For this review, take the finished solid that the model builds, in its own axes (mm). A direction names the side the tool comes from. Give positions to 0.01 mm unless a question says otherwise; leave off trailing zeros. Write each loop counter-clockwise with the first axis right and the second up, starting at its lowest first coordinate (ties: lowest second). Pieces come first, ordered by that corner, then holes. Notation, with made-up numbers: (2, 55) -> (57, 55) arc R25 cw to (57, 72) -> close; hole circle Ø4 at (22.25, 71.25). An arc over 180 degrees is marked (long way). Answer as CSV lines item,"result".
```python
from build123d import *

# Parameters (mm, degrees)
SKETCH2_R           = 31.5
SKETCH2_R_2         = 7.5
BOSS_EXTRUDE1_DEPTH = 7.55
SKETCH4_R           = 13.75
SKETCH4_R_2         = 7.5
BOSS_EXTRUDE2_DEPTH = 7.45
CUT_EXTRUDE1_DEPTH  = 48.005318848


with BuildPart() as part:
    # Sketch2 → Boss-Extrude1 (new body)
    with BuildSketch(Plane.XY):
        Circle(SKETCH2_R)
        Circle(SKETCH2_R_2, mode=Mode.SUBTRACT)
    extrude(amount=BOSS_EXTRUDE1_DEPTH)

    # Sketch4 → Boss-Extrude2 (add)
    with BuildSketch(Plane.XY.offset(7.55)):
        Circle(SKETCH4_R)
        Circle(SKETCH4_R_2, mode=Mode.SUBTRACT)
    extrude(amount=BOSS_EXTRUDE2_DEPTH)

    # Sketch5 → Cut-Extrude1 (cut, through all)
    with BuildSketch(Plane.XY.offset(15)):
        with BuildLine():
            Line((2.5, 9.8), (-2.5, 9.8))
            Line((-2.5, 9.8), (-2.5, 7.071067812))
            ThreePointArc((-2.5, 7.071067812), (0, 7.5), (2.5, 7.071067812))
            Line((2.5, 7.071067812), (2.5, 9.8))
        make_face()
    extrude(amount=-CUT_EXTRUDE1_DEPTH, mode=Mode.SUBTRACT)


solid = part.part
```
Q1. Add section D-D (y = -13). Write out the cut boundary in (x, z), plus the area to 3 significant figures.
Answer block:
outline,"(-28.69, 0) -> (28.69, 0) -> (28.69, 7.55) -> (4.48, 7.55) -> (4.48, 15) -> (-4.48, 15) -> (-4.48, 7.55) -> (-28.69, 7.55) -> close"
area,"500 mm2"
Q2. Draft analysis for pull direction Y (two halves, no side actions). For faces 4 (the flat face through (14, -7, 7.55)), 5 (the cylindrical face through (-0.294, -7.494, 7.395)), 6 (the cylindrical face through (-4.101, 31.232, 3.722)), 7 (the flat face through (-2.5, 8, 8)), state which applies: released by +Y, released by -Y, zero draft, split by the parting line, or undercut.
Answer block:
face 4,"zero draft"
face 5,"undercut"
face 6,"split by the parting line"
face 7,"undercut"
Q3. For faces 1 (the flat face through (6, -6, 15)), 2 (the cylindrical face through (-2.981, -13.423, 11.223)), 3 (the flat face through (2.5, 8, 8)), list the 3-axis set-ups (+Z, -Z, +X, -X, +Y, -Y) from which the entire face can be reached by the end or side of a thin tool; tool diameter is ignored.
Answer block:
face 1,"+Z, +X, -X, +Y, -Y"
face 2,"+Z"
face 3,"+Z, -Z"
Q4. Clearance check with flat-ended pins moving along their axes: pin 1 (1 mm diameter, centred on y = -9, z = 12.5, fed in from -X); pin 2 (9 mm diameter, centred on x = 0, y = 0, fed in from +Z); pin 3 (3 mm diameter, centred on y = 8.5, z = 4.5, fed in from -X); pin 4 (5 mm diameter, centred on x = 3, z = 8, fed in from +Y). State where each tip first meets the part, or that it passes through.
Answer block:
pin 1,"stops at x = -10.81"
pin 2,"passes through"
pin 3,"stops at x = -30.71"
pin 4,"stops at y = 31.5"
Q5. Add section C-C (z = 3). Write out the cut boundary in (x, y), plus the area to 3 significant figures.
Answer block:
outline,"circle Ø63 at (0, 0); hole (-2.5, 7.07) arc R7.5 ccw (long way) to (2.5, 7.07) -> (2.5, 9.8) -> (-2.5, 9.8) -> close"
area,"2,930 mm2"
Q6. To check wall thickness, follow probe 1 along Y at (x, z) = (0, 5.75); probe 2 along Z at (x, y) = (-12.5, 10); probe 3 along X at (y, z) = (6, 5.5). State the ranges of each line that lie inside material, in increasing order. Write a range as [from, to].
Answer block:
probe 1,"y = [-31.5, -7.5], [9.8, 31.5]"
probe 2,"z = [0, 7.55]"
probe 3,"x = [-30.92, -4.5], [4.5, 30.92]"
Q7. Add section B-B (x = 0). Write out the cut boundary in (y, z), plus the area to 3 significant figures.
Answer block:
outline,"(-31.5, 0) -> (-7.5, 0) -> (-7.5, 15) -> (-13.75, 15) -> (-13.75, 7.55) -> (-31.5, 7.55) -> close; (9.8, 0) -> (31.5, 0) -> (31.5, 7.55) -> (13.75, 7.55) -> (13.75, 15) -> (9.8, 15) -> close"
area,"421 mm2"
Q8. Add section A-A (y = 0). Write out the cut boundary in (x, z), plus the area to 3 significant figures.
Answer block:
outline,"(-31.5, 0) -> (-7.5, 0) -> (-7.5, 15) -> (-13.75, 15) -> (-13.75, 7.55) -> (-31.5, 7.55) -> close; (7.5, 0) -> (31.5, 0) -> (31.5, 7.55) -> (13.75, 7.55) -> (13.75, 15) -> (7.5, 15) -> close"
area,"456 mm2"
